```python
from build123d import *

# Parameters (mm, degrees)
F0_R     = 34.003595
F1_DEPTH = 3
F2_R     = 30.383163
F3_DEPTH = 2.54
F5_DEPTH = 25.4


with BuildPart() as f1:
    # F0 (on Front) → F1 (new body)
    with BuildSketch(Plane.XZ):
        Circle(F0_R)
    extrude(amount=F1_DEPTH)

    # F2 (on face) → F3 (join)
    with BuildSketch(Plane.XZ.offset(3)):
        Circle(F2_R)
    extrude(amount=F3_DEPTH)

    # F4 (on face) → F5 (cut)
    with BuildSketch(Plane(origin=(0, 0, 0), x_dir=(-1, 0, 0), z_dir=(0, 1, 0))):
        with BuildLine():
            Line((-1.27, 0), (0, 0))
            Line((0, 0), (1.27, 0))
            Line((1.27, 0), (1.27, 33.97987))
            ThreePointArc((1.27, 33.97987), (0, 34.003595), (-1.27, 33.97987))
            Line((-1.27, 33.97987), (-1.27, 0))
        make_face()
    extrude(amount=-F5_DEPTH, mode=Mode.SUBTRACT)


solid = f1.part
```
Model file for the job. Use its own axes, mm. A direction names the side the tool comes from. Give positions to 0.01 mm unless a question says otherwise; leave off trailing zeros. Loops run counter-clockwise (first coordinate to the right, second up) from the corner with the lowest first, then second, coordinate; pieces in that order, holes last. Notation, with made-up numbers: (48, -27.75) -> (104, -27.75) arc R18 cw to (104, -10.75) -> close; hole circle Ø2 at (50.25, 60). An arc over 180 degrees is marked (long way). Use CSV: the item, a comma, the result in double quotes. Start each with the question number.
1) Flat gauge pins, fed straight in: pin 1 Ø1 at (x, y) = (-5, -4) entering from -Z; pin 2 Ø3 at (y, z) = (-3.5, 23) entering from -X; pin 3 Ø3 at (x, y) = (2.5, -2) entering from -Z; pin 4 Ø6 at (x, z) = (-6, 6) entering from +Y. Where does each tip first touch, or does it go through?
2) Wall check: line 1 (X direction, y = -2.55, z = 9.5); line 2 (X direction, y = -4, z = 17); line 3 (Y direction, x = 23, z = -21). Give the ranges that are in metal, low to high.
3) Slice it at D-D on x = 21. Give the cut face in (y, z).
4) Tool access for faces 4 (the flat face through (1.27, -3, 17)), 5 (the flat face through (0, -5.54, -6)), 6 (the flat face through (-5.2, -3, 30.4)): list every direction of +Z, -Z, +X, -X, +Y, -Y with a clear straight run to the whole face (end or side of a thin tool).
5) Slice it at A-A on z = 26.5. Give the cut face in (x, y), plus the area to 3 significant figures.
6) Slice it at C-C on y = -4.35. Give the cut face in (x, z), plus the area to 3 significant figures.
7) Mould opens along X. For faces 1 (the flat face through (-1.27, -3, 17)), 2 (the flat face through (0, -3, 0)), 3 (the flat face through (0, 0, -7)) say: released by +X, released by -X, zero draft, split by the parting line, or undercut.
8) Slice it at B-B on x = 0. Give the cut face in (y, z), plus the area to 3 significant figures.
Computed values:
1,pin 1,"stops at z = -30.05"
1,pin 2,"stops at x = -26.27"
1,pin 3,"stops at z = -33.99"
1,pin 4,"stops at y = 0"
2,line 1,"x = -32.65 to -1.27, 1.27 to 32.65"
2,line 2,"x = -25.18 to -1.27, 1.27 to 25.18"
2,line 3,"y = -3 to 0"
3,outline,"(-5.54, -21.96) -> (-3, -21.96) -> (-3, -26.74) -> (0, -26.74) -> (0, 26.74) -> (-3, 26.74) -> (-3, 21.96) -> (-5.54, 21.96) -> close"
4,face 4,"+Z, +Y, -Y"
4,face 5,"+Z, -Z, +X, -X, -Y"
4,face 6,"-Y"
5,outline,"(-21.31, -3) -> (-14.86, -3) -> (-14.86, -5.54) -> (-1.27, -5.54) -> (-1.27, 0) -> (-21.31, 0) -> close; (1.27, -5.54) -> (14.86, -5.54) -> (14.86, -3) -> (21.31, -3) -> (21.31, 0) -> (1.27, 0) -> close"
5,area,"189 mm^2"
6,outline,"(-1.27, 0) -> (-1.27, 30.36) arc R30.38 ccw (long way) to (1.27, 30.36) -> (1.27, 0) -> close"
6,area,"2,820 mm^2"
7,face 1,"undercut"
7,face 2,"undercut"
7,face 3,"zero draft"
8,outline,"(-5.54, -30.38) -> (-3, -30.38) -> (-3, -34) -> (0, -34) -> (0, 0) -> (-5.54, 0) -> close"
8,area,"179 mm^2"
